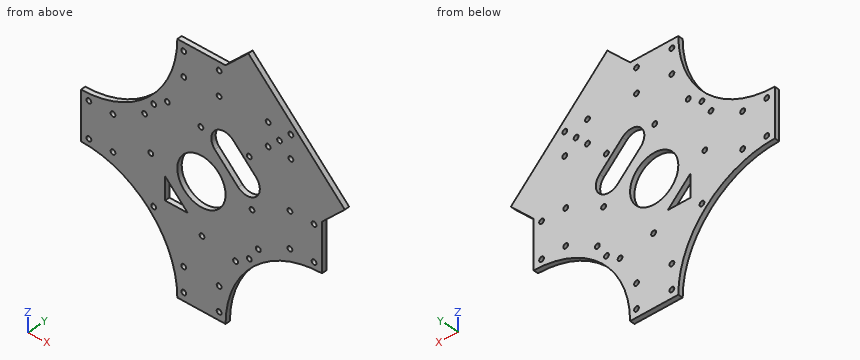
from build123d import *

# Parameters (mm, degrees)
SKETCH_1_R           = 1.25
EXTRUDE_1_DEPTH      = 3
SKETCH_2_R           = 1.5
CUT_EXTRUDE_1_DEPTH  = 3
CUT_EXTRUDE_2_DEPTH  = 3
CUT_EXTRUDE_3_DEPTH  = 3
CUT_EXTRUDE_4_DEPTH  = 10
SKETCH_6_R           = 1.5
CUT_EXTRUDE_5_DEPTH  = 10
SKETCH_7_R           = 1.5
CUT_EXTRUDE_8_DEPTH  = 10
SKETCH_8_R           = 1.5
CUT_EXTRUDE_9_DEPTH  = 10
SKETCH_9_R           = 15
CUT_EXTRUDE_10_DEPTH = 10
EXTRUDE_START        = -3
EXTRUDE_2_DEPTH      = 3
SKETCH_11_R          = 1.5
CUT_EXTRUDE_11_DEPTH = 3
SKETCH_12_R          = 1.5
CUT_EXTRUDE_12_DEPTH = 3


with BuildPart() as part:
    # 草图1 → 凸台-拉伸1 (new body)
    # profile 1 of 4: a face of its own
    with BuildSketch(Plane(origin=(0, 0, 0), x_dir=(1, 0, 0), z_dir=(0, 1, 0))):
        with BuildLine():
            ThreePointArc((75, -15), (32.573593129, -32.573593129), (15, -75))
            Line((15, -75), (0, -75))
            Line((0, -75), (0, 0))
            Line((0, 0), (75, 0))
            Line((75, 0), (75, -15))
        make_face()
        with Locations(Location((11, -70, 0), (0, 0, 270))):
            Circle(SKETCH_1_R, mode=Mode.SUBTRACT)
        with Locations(Location((70, -11, 0), (0, 0, 270))):
            Circle(SKETCH_1_R, mode=Mode.SUBTRACT)
    # profile 2 of 4: a face of its own
    with BuildSketch(Plane(origin=(0, 0, 0), x_dir=(1, 0, 0), z_dir=(0, 1, 0))):
        with BuildLine():
            ThreePointArc((-15, -75), (-32.573593129, -32.573593129), (-75, -15))
            Line((-75, -15), (-75, 0))
            Line((-75, 0), (0, 0))
            Line((0, 0), (0, -75))
            Line((0, -75), (-15, -75))
        make_face()
        with Locations(Location((-70, -11, 0), (0, 0, 270))):
            Circle(SKETCH_1_R, mode=Mode.SUBTRACT)
        with Locations(Location((-11, -70, 0), (0, 0, 270))):
            Circle(SKETCH_1_R, mode=Mode.SUBTRACT)
    # profile 3 of 4: a face of its own
    with BuildSketch(Plane(origin=(0, 0, 0), x_dir=(1, 0, 0), z_dir=(0, 1, 0))):
        with BuildLine():
            ThreePointArc((-75, 15), (-32.573593129, 32.573593129), (-15, 75))
            Line((-15, 75), (0, 75))
            Line((0, 75), (0, 0))
            Line((0, 0), (-75, 0))
            Line((-75, 0), (-75, 15))
        make_face()
        with Locations(Location((-11, 70, 0), (0, 0, 270))):
            Circle(SKETCH_1_R, mode=Mode.SUBTRACT)
        with Locations(Location((-70, 11, 0), (0, 0, 270))):
            Circle(SKETCH_1_R, mode=Mode.SUBTRACT)
    # profile 4 of 4: a face of its own
    with BuildSketch(Plane(origin=(0, 0, 0), x_dir=(1, 0, 0), z_dir=(0, 1, 0))):
        with BuildLine():
            ThreePointArc((15, 75), (32.573593129, 32.573593129), (75, 15))
            Line((75, 15), (75, 0))
            Line((75, 0), (0, 0))
            Line((0, 0), (0, 75))
            Line((0, 75), (15, 75))
        make_face()
        with Locations(Location((70, 11, 0), (0, 0, 270))):
            Circle(SKETCH_1_R, mode=Mode.SUBTRACT)
        with Locations(Location((11, 70, 0), (0, 0, 270))):
            Circle(SKETCH_1_R, mode=Mode.SUBTRACT)
    extrude(amount=EXTRUDE_1_DEPTH)

    # 草图2 → 切除-拉伸1 (cut)
    with BuildSketch(Plane.XZ):
        with Locations(Location((0.353553391, -31.466251763, 0), (0, 0, 270))):
            Circle(SKETCH_2_R)
        with Locations(Location((31.466251763, -0.353553391, 0), (0, 0, 270))):
            Circle(SKETCH_2_R)
        with Locations(Location((-0.353553391, 31.466251763, 0), (0, 0, 90))):
            Circle(SKETCH_2_R)
        with Locations(Location((-31.466251763, 0.353553391, 0), (0, 0, 90))):
            Circle(SKETCH_2_R)
    extrude(amount=-CUT_EXTRUDE_1_DEPTH, mode=Mode.SUBTRACT)

    # 草图3 → 切除-拉伸2 (cut)
    with BuildSketch(Plane(origin=(0, 3, 0), x_dir=(1, 0, 0), z_dir=(0, 1, 0))):
        Polygon((-15.556349186, 15.556349186), (-12.02081528, 19.091883092), (-22.627416998, 22.627416998), align=None)
        Polygon((-19.091883092, 12.02081528), (-15.556349186, 15.556349186), (-22.627416998, 22.627416998), align=None)
    extrude(amount=-CUT_EXTRUDE_2_DEPTH, mode=Mode.SUBTRACT)

    # 草图4 → 切除-拉伸3 (cut)
    with BuildSketch(Plane(origin=(0, 3, 0), x_dir=(1, 0, 0), z_dir=(0, 1, 0))):
        with BuildLine():
            ThreePointArc((33.944668714, -19.80253309), (34.043922781, -8.582763971), (22.827665534, -8.285032838))
            Line((22.827665534, -8.285032838), (15.556349186, -15.556349186))
            Line((15.556349186, -15.556349186), (8.285032838, -22.827665534))
            ThreePointArc((8.285032838, -22.827665534), (8.582763971, -34.043922781), (19.80253309, -33.944668714))
            Line((19.80253309, -33.944668714), (33.944668714, -19.80253309))
        make_face()
    extrude(amount=-CUT_EXTRUDE_3_DEPTH, mode=Mode.SUBTRACT)

    # 草图5 → 切除-拉伸4 (cut)
    with BuildSketch(Plane(origin=(0, 3, 0), x_dir=(1, 0, 0), z_dir=(0, 1, 0))):
        Polygon((-22.627416998, 8.485281374), (-22.627416998, 22.627416998), (-19.091883092, 12.02081528), align=None)
        Polygon((-12.02081528, 19.091883092), (-22.627416998, 22.627416998), (-8.485281374, 22.627416998), align=None)
    extrude(amount=-CUT_EXTRUDE_4_DEPTH, mode=Mode.SUBTRACT)

    # 草图6 → 切除-拉伸5 (cut)
    with BuildSketch(Plane(origin=(0, 3, 0), x_dir=(1, 0, 0), z_dir=(0, 1, 0))):
        with Locations(Location((-35.355339059, -21.213203436, 0), (0, 0, 270))):
            Circle(SKETCH_6_R)
        with Locations(Location((-21.213203436, -35.355339059, 0), (0, 0, 270))):
            Circle(SKETCH_6_R)
        with Locations(Location((35.355339059, 21.213203436, 0), (0, 0, 270))):
            Circle(SKETCH_6_R)
        with Locations(Location((21.213203436, 35.355339059, 0), (0, 0, 270))):
            Circle(SKETCH_6_R)
    extrude(amount=-CUT_EXTRUDE_5_DEPTH, mode=Mode.SUBTRACT)

    # 草图7 → 切除-拉伸8 (cut)
    with BuildSketch(Plane(origin=(0, 3, 0), x_dir=(1, 0, 0), z_dir=(0, 1, 0))):
        with Locations(Location((-29.69848481, 29.69848481, 0), (0, 0, 270))):
            Circle(SKETCH_7_R)
        with Locations(Location((29.69848481, 29.69848481, 0), (0, 0, 270))):
            Circle(SKETCH_7_R)
        with Locations(Location((29.69848481, -29.69848481, 0), (0, 0, 270))):
            Circle(SKETCH_7_R)
        with Locations(Location((-29.69848481, -29.69848481, 0), (0, 0, 270))):
            Circle(SKETCH_7_R)
    extrude(amount=-CUT_EXTRUDE_8_DEPTH, mode=Mode.SUBTRACT)

    # 草图8 → 切除-拉伸9 (cut)
    with BuildSketch(Plane(origin=(0, 3, 0), x_dir=(1, 0, 0), z_dir=(0, 1, 0))):
        with Locations(Location((-11, 55, 0), (0, 0, 270))):
            Circle(SKETCH_8_R)
        with Locations(Location((11, 55, 0), (0, 0, 270))):
            Circle(SKETCH_8_R)
        with Locations(Location((55, 11, 0), (0, 0, 270))):
            Circle(SKETCH_8_R)
        with Locations(Location((55, -11, 0), (0, 0, 270))):
            Circle(SKETCH_8_R)
        with Locations(Location((11, -55, 0), (0, 0, 270))):
            Circle(SKETCH_8_R)
        with Locations(Location((-11, -55, 0), (0, 0, 270))):
            Circle(SKETCH_8_R)
        with Locations(Location((-55, -11, 0), (0, 0, 270))):
            Circle(SKETCH_8_R)
        with Locations(Location((-55, 11, 0), (0, 0, 270))):
            Circle(SKETCH_8_R)
    extrude(amount=-CUT_EXTRUDE_9_DEPTH, mode=Mode.SUBTRACT)

    # 草图9 → 切除-拉伸10 (cut)
    with BuildSketch(Plane(origin=(0, 3, 0), x_dir=(1, 0, 0), z_dir=(0, 1, 0))):
        with Locations(Location((0, 0, 0), (0, 0, 270))):
            Circle(SKETCH_9_R)
    extrude(amount=-CUT_EXTRUDE_10_DEPTH, mode=Mode.SUBTRACT)

    # 草图10 → 凸台-拉伸2 (add)
    with BuildSketch(Plane(origin=(0, 3, 0), x_dir=(1, 0, 0), z_dir=(0, 1, 0)).offset(EXTRUDE_START)):
        Polygon((89.142135624, -29.142135624), (29.142135624, -89.142135624), (15, -75), (75, -15), align=None)
        with BuildLine():
            Line((75, -15), (15, -75))
            ThreePointArc((15, -75), (32.573593129, -32.573593129), (75, -15))
        make_face()
    extrude(amount=EXTRUDE_2_DEPTH)

    # 草图11 → 切除-拉伸11 (cut)
    with BuildSketch(Plane(origin=(0, 3, 0), x_dir=(1, 0, 0), z_dir=(0, 1, 0))):
        with Locations(Location((11, 70, 0), (0, 0, 270))):
            Circle(SKETCH_11_R)
        with Locations(Location((-11, 70, 0), (0, 0, 270))):
            Circle(SKETCH_11_R)
        with Locations(Location((70, 11, 0), (0, 0, 270))):
            Circle(SKETCH_11_R)
        with Locations(Location((70, -11, 0), (0, 0, 270))):
            Circle(SKETCH_11_R)
        with Locations(Location((11, -70, 0), (0, 0, 270))):
            Circle(SKETCH_11_R)
        with Locations(Location((-11, -70, 0), (0, 0, 270))):
            Circle(SKETCH_11_R)
        with Locations(Location((-70, -11, 0), (0, 0, 270))):
            Circle(SKETCH_11_R)
        with Locations(Location((-70, 11, 0), (0, 0, 270))):
            Circle(SKETCH_11_R)
    extrude(amount=-CUT_EXTRUDE_11_DEPTH, mode=Mode.SUBTRACT)

    # 草图12 → 切除-拉伸12 (cut)
    with BuildSketch(Plane(origin=(0, 3, 0), x_dir=(1, 0, 0), z_dir=(0, 1, 0))):
        with Locations(Location((48.535533906, -48.535533906, 0), (0, 0, 270))):
            Circle(SKETCH_12_R)
        with Locations(Location((55.606601718, -41.464466094, 0), (0, 0, 270))):
            Circle(SKETCH_12_R)
        with Locations(Location((55.606601718, -55.606601718, 0), (0, 0, 270))):
            Circle(SKETCH_12_R)
        with Locations(Location((41.464466094, -55.606601718, 0), (0, 0, 270))):
            Circle(SKETCH_12_R)
        with Locations(Location((41.464466094, -41.464466094, 0), (0, 0, 270))):
            Circle(SKETCH_12_R)
    extrude(amount=-CUT_EXTRUDE_12_DEPTH, mode=Mode.SUBTRACT)


solid = part.part
Geometry check sheet. Reference: the model listing, model coordinates, mm. Coordinates: 2 decimals unless noted, no trailing zeros. Order: outer loops, then holes, each group sorted by start corner. A loop starts at its lowest first (then second) coordinate and runs counter-clockwise, first axis right, second up. Notation, with made-up numbers: (72, 43) - (108, 43) arc R10 cw to (108, 59) - close; hole circle Ø8 at (47.5, 38). An arc over 180 degrees is marked (long way). Answer in a Markdown table with one row per item. Add a question column.
1) Cross-section at B-B, the plane y = 2.05. State how many separate pieces and enclosed holes the cut face has, then the cut area to 3 significant figures.
2) Cross-section at C-C, the plane z = -41. Record the cut outline in (x, y).
3) Material ranges on line 1 along X through (y, z) = (2.45, 22.5); line 2 along X through (y, z) = (1.25, -1.5); line 3 along Z through (x, y) = (-22, 1.75), recorded low to high. Write a range as [from, to].
4) Gauge pin test, flat end, axial feed: P1, Ø1.8, axis at x = 11, z = 55, coming from the +Y side. Record the tip position at first contact, or that the pin passes through.
5) Cross-section at A-A, the plane x = -46. Record the cut outline in (y, z), then the cut area to 3 significant figures.
Check result:
| question | item | result |
|---|---|---|
| 1 | separate pieces | 1 |
| 1 | enclosed holes | 36 |
| 1 | area | 12,400 mm² |
| 2 | outline | (-25.56, 0) - (25.56, 0) - (25.56, 3) - (-25.56, 3) - close |
| 3 | line 1 | x = [-45.95, -36.13], [-34.58, 8.61], [31.25, 82.5] |
| 3 | line 2 | x = [-75, -14.92], [14.92, 30.5], [32.43, 75] |
| 3 | line 3 | z = [-46.88, -22.63], [-9.11, 34.08], [36.63, 46.88] |
| 4 | P1 | passes through |
| 5 | outline | (0, -22.47) - (3, -22.47) - (3, 22.47) - (0, 22.47) - close |
| 5 | area | 135 mm² |
